Drawing for the job (mm, zero at the part's lowest x, y, z). A direction names the side the tool comes from. Round coordinates to 2 decimals unless told otherwise and drop trailing zeros. Order: outer loops, then holes, each group sorted by start corner. A loop starts at its lowest first (then second) coordinate and runs counter-clockwise, first axis right, second up. Notation, with made-up numbers: (-2.5, 66.25) - (36.5, 66.25) arc R29 cw to (36.5, 91.25) - close; hole circle Ø11 at (62, -25). An arc over 180 degrees is marked (long way). One line per question, with ' | ' between items. Start each with the question number.
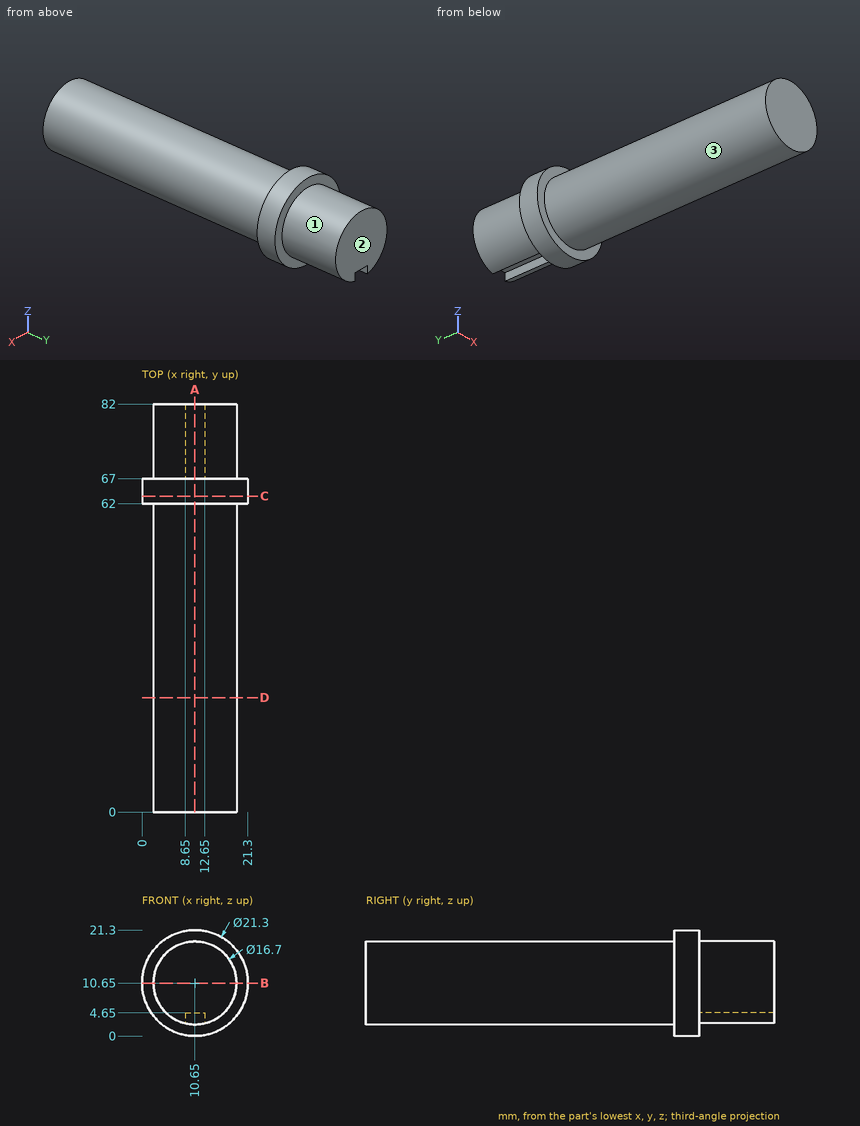
Item 1: Slice it at D-D (y = 23). Write the cut outline in (x, z).
Item 2: Pin check, flat tips, straight feed: pin 1 (10 mm diameter, centred on y = 17, z = 8, fed in from -X); pin 2 (4 mm diameter, centred on y = 48, z = 14.5, fed in from +X); pin 3 (1 mm diameter, centred on y = 54.5, z = 17.5, fed in from -X). Stop position of each tip, or through.
Item 3: Wall check: line 1 along Y through (x, z) = (8.75, 20); line 2 along Y through (x, z) = (12, 2.75); line 3 along Z through (x, y) = (9.75, 65). Give the ranges that are in metal, low to high. Write a range as [from, to].
Item 4: Slice it at B-B (z = 10.65). Write the cut outline in (x, y).
Item 5: 3-axis set-ups, long thin cutter, end or side, ignore diameter. For the marked faces 1, 2 and 3: which of +Z, -Z, +X, -X, +Y, -Y reach the whole face in a straight line?
Item 6: Slice it at A-A (x = 10.65). Write the cut outline in (y, z), plus the area to 3 significant figures.
Item 7: Slice it at C-C (y = 63.5). Write the cut outline in (x, z).
A:
1) outline: circle Ø16.7 at (10.65, 10.65)
2) pin 1: x = 2.3 | pin 2: x = 18.79 | pin 3: x = 5.23
3) line 1: [62, 67] | line 2: [0, 67] | line 3: [0.04, 21.26]
4) outline: (0, 62) - (2.3, 62) - (2.3, 0) - (19, 0) - (19, 62) - (21.3, 62) - (21.3, 67) - (19, 67) - (19, 82) - (2.3, 82) - (2.3, 67) - (0, 67) - close
5) face 1: +Y | face 2: +Z, -Z, +X, -X, +Y | face 3: -Y
6) outline: (0, 2.3) - (62, 2.3) - (62, 0) - (67, 0) - (67, 4.65) - (82, 4.65) - (82, 19) - (67, 19) - (67, 21.3) - (62, 21.3) - (62, 19) - (0, 19) - close | area: 1,360 mm^2
7) outline: circle Ø21.3 at (10.65, 10.65)
